Input: dimensioned drawing with shaded views. Units: mm. Origin: part minimum x, y, z. A direction names the side the tool comes from. Coordinates: 2 decimals unless noted, no trailing zeros. Loops run counter-clockwise (first coordinate to the right, second up) from the corner with the lowest first, then second, coordinate; pieces in that order, holes last.
(1) Contact query for flat-ended pins moving along their axis: P1, Ø10, axis at y = 18.5, z = 7, coming from the +X side (1 decimal); P2, Ø10, axis at x = 17, z = 24.5, coming from the +Y side; P3, Ø4, axis at x = 71, y = 22, coming from the +Z side; P4, Ø7, axis at x = 38.1, z = 38.1, coming from the +Y side. Output: stop coordinate, or through.
(2) Set-up query: the marked faces 1, 2 and 3. Return all of +Z, -Z, +X, -X, +Y, -Y with unobstructed straight access to the full face (end or side cutting, diameter ignored); none if empty.
(3) Mould query, pull axis X, two halves, no side actions, for the marked faces 4, 5 and 6. Classes: released by +X, released by -X, zero draft, split by the parting line, or undercut.
(4) Line query: L1, parallel to Z at x = 38.1, y = 8.5; L2, parallel to Z at x = 38.1, y = 1.4. Output: solid intervals per line, ascending.
(5) Section A-A, the plane z = 37. Return loops of the section in (x, y), then the cut area to 3 significant figures.
(6) Section C-C, the plane z = 45.5. Return loops of the section in (x, y) (1 decimal), then the cut area to 3 significant figures.
(7) Section D-D, the plane x = 27. Return loops of the section in (y, z).
(8) Section B-B, the plane y = 4.75. Return loops of the section in (x, z), then the cut area to 3 significant figures.
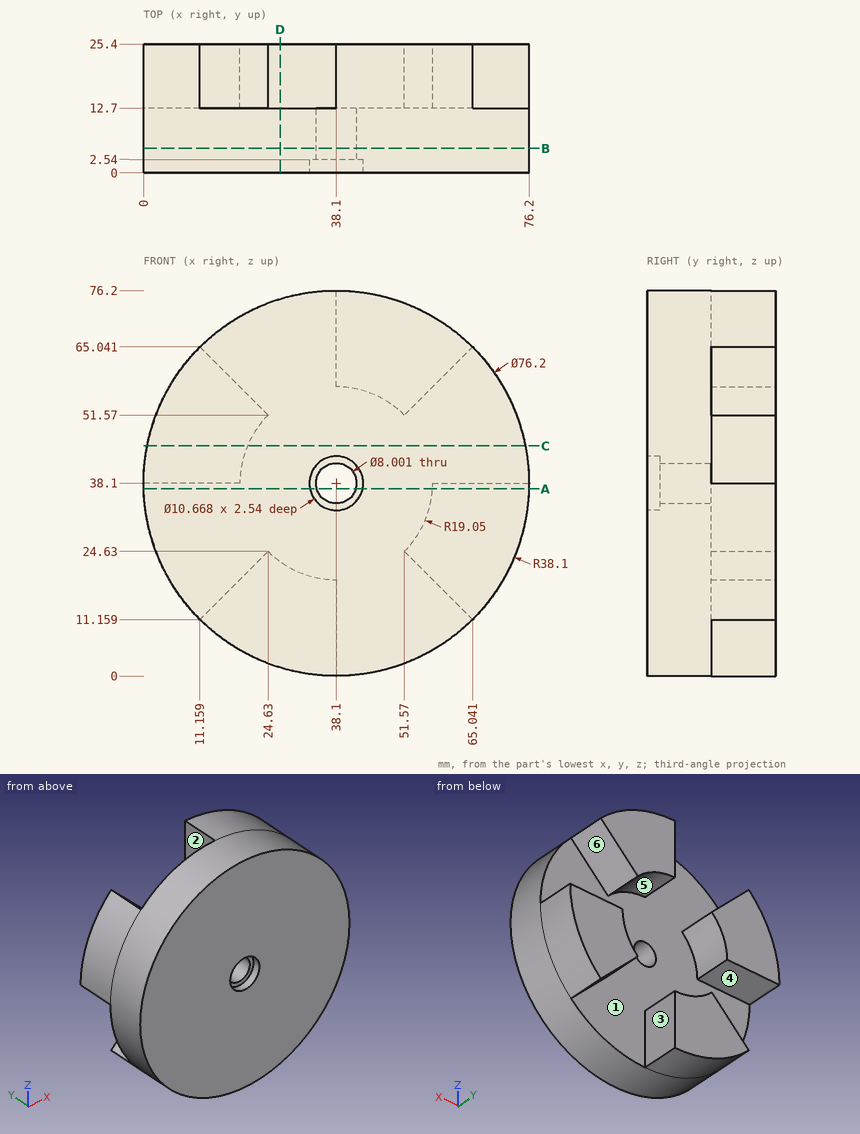
Report:
1. P1: stops at x = 65.9
1. P2: stops at y = 12.7
1. P3: stops at z = 38.1
1. P4: passes through
2. face 1: +Y
2. face 2: +Z, +Y
2. face 3: -Z, +Y
3. face 4: zero draft
3. face 5: undercut
3. face 6: released by +X
4. L1: z = 0 to 34.1, 42.1 to 76.2
4. L2: z = 0 to 32.77, 43.43 to 76.2
5. outline: (0.02, 0) - (32.88, 0) - (32.88, 2.54) - (34.25, 2.54) - (34.25, 12.7) - (0.02, 12.7) - close; (41.95, 2.54) - (43.32, 2.54) - (43.32, 0) - (76.18, 0) - (76.18, 25.4) - (57.12, 25.4) - (57.12, 12.7) - (41.95, 12.7) - close
5. area: 1,100 mm2
6. outline: (0.7, 0) - (75.5, 0) - (75.5, 12.7) - (20.5, 12.7) - (20.5, 25.4) - (0.7, 25.4) - close
6. area: 1,200 mm2
7. outline: (0, 1.65) - (25.4, 1.65) - (25.4, 22.62) - (12.7, 22.62) - (12.7, 74.55) - (0, 74.55) - close
8. outline: circle Ø76.2 at (38.1, 38.1); hole circle Ø8 at (38.1, 38.1)
8. area: 4,510 mm2
